Source: CAD feature listing. Evaluate the final solid. Frame: model axes, mm. Face numbers are marked on the shaded views. A direction names the side the tool comes from. Coordinates: 2 decimals unless noted, no trailing zeros. Order: outer loops, then holes, each group sorted by start corner. A loop starts at its lowest first (then second) coordinate and runs counter-clockwise, first axis right, second up. Notation, with made-up numbers: (60, 68.5) - (67, 68.5) arc R27 cw to (67, 87.5) - close; hole circle Ø5 at (-11.75, 35). An arc over 180 degrees is marked (long way). One line per question, with ' | ' between items.
from build123d import *

# Parameters (mm, degrees)
F0_W     = 30
F0_H     = 31
F1_DEPTH = 2.5
F2_R     = 1.5
F3_DEPTH = 2.501
F4_W     = 31
F4_H     = 14.5
F5_DEPTH = 2.5
F6_R     = 2.5
F7_DEPTH = 32.501


with BuildPart() as f1:
    # F0 (on Top) → F1 (new body)
    with BuildSketch(Plane.XY):
        Rectangle(F0_W, F0_H)
    extrude(amount=F1_DEPTH)

    # F2 (on face) → F3 (cut, through all)
    with BuildSketch(Plane.XY.offset(2.5)):
        with Locations((-12, -12)):
            Circle(F2_R)
        with Locations((8, -12)):
            Circle(F2_R)
        with Locations((8, 12)):
            Circle(F2_R)
    extrude(amount=-F3_DEPTH, mode=Mode.SUBTRACT)

    # F4 (on face) → F5 (join)
    with BuildSketch(Plane.YZ.offset(15)):
        with Locations((0, 7.25)):
            Rectangle(F4_W, F4_H)
    extrude(amount=F5_DEPTH)

    # F6 (on face) → F7 (cut, through all)
    with BuildSketch(Plane.YZ.offset(17.5)):
        with Locations((0, 8.5)):
            Circle(F6_R)
    extrude(amount=-F7_DEPTH, mode=Mode.SUBTRACT)


solid = f1.part
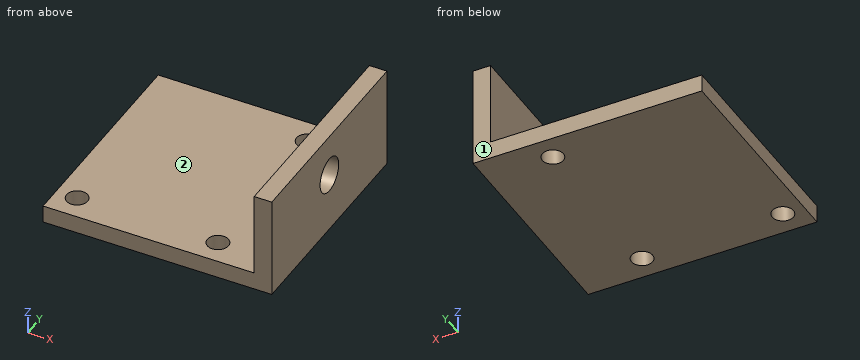
(1) Cut plane B-B (y = -12). Return the cut outline in (x, z).
Taken from the geometry:
outline: (-15, 0) - (-13.5, 0) - (-13.5, 2.5) - (-15, 2.5) - close; (-10.5, 0) - (6.5, 0) - (6.5, 2.5) - (-10.5, 2.5) - close; (9.5, 0) - (17.5, 0) - (17.5, 14.5) - (15, 14.5) - (15, 2.5) - (9.5, 2.5) - close
(2) Set-up query: the marked faces 1 and 2. Return all of +Z, -Z, +X, -X, +Y, -Y with unobstructed straight access to the full face (end or side cutting, diameter ignored); none if empty.
Taken from the geometry:
face 1: +Z, -Z, +X, -X, +Y | face 2: +Z, -X, +Y, -Y
(3) Material intervals for L1, parallel to Y at x = 8, z = 0.85; L2, parallel to Y at x = -12, z = 1.75; L3, parallel to X at y = -11, z = 2, sorted ascending. Write a range as from..to.
Taken from the geometry:
L1: y = -15.5..-13.5, -10.5..10.5, 13.5..15.5 | L2: y = -15.5..-13.5, -10.5..15.5 | L3: x = -15..-13.12, -10.88..6.88, 9.12..17.5
(4) Cut plane D-D (y = 2). Return the cut outline in (x, z), and give its area (3 significant figures).
Taken from the geometry:
outline: (-15, 0) - (17.5, 0) - (17.5, 7) - (15, 7) - (15, 2.5) - (-15, 2.5) - close; (15, 10) - (17.5, 10) - (17.5, 14.5) - (15, 14.5) - close | area: 104 mm²
(5) Cut plane A-A (x = 8). Return the cut outline in (y, z).
Taken from the geometry:
outline: (-15.5, 0) - (-13.5, 0) - (-13.5, 2.5) - (-15.5, 2.5) - close; (-10.5, 0) - (10.5, 0) - (10.5, 2.5) - (-10.5, 2.5) - close; (13.5, 0) - (15.5, 0) - (15.5, 2.5) - (13.5, 2.5) - close
(6) Cut plane C-C (x = -12). Return the cut outline in (y, z).
Taken from the geometry:
outline: (-15.5, 0) - (-13.5, 0) - (-13.5, 2.5) - (-15.5, 2.5) - close; (-10.5, 0) - (15.5, 0) - (15.5, 2.5) - (-10.5, 2.5) - close
(7) Pin query (flat end, axial travel): P1, Ø1.8, axis at x = 8, y = -12, coming from the +Z side; P2, Ø6, axis at y = 4, z = 8, coming from the -X side; P3, Ø15, axis at x = -0.5, y = -2, coming from the +Z side; P4, Ø8, axis at x = 12, z = 6, coming from the -Y side. Return the tip coordinate at first contact, or that it passes through.
Taken from the geometry:
P1: passes through | P2: stops at x = 15 | P3: stops at z = 2.5 | P4: stops at y = -15.5
